from build123d import *

# Parameters (mm, degrees)
CYLINDER015_R     = 4.5
CYLINDER015_DEPTH = 4.6
CYLINDER014_R     = 6
CYLINDER014_DEPTH = 4.6
CYLINDER013_W     = 6
CYLINDER013_H     = 5
CYLINDER013_ANGLE = 39
CYLINDER012_W     = 7
CYLINDER012_H     = 5
CYLINDER012_ANGLE = 39
CHAMFER007_SIZE   = 0.2
ARRAY001_COUNT    = 9


with BuildPart() as cilindro011:
    # Cylinder015 → Cylinder015 (new body)
    with BuildSketch(Plane.XY.offset(0.2)):
        Circle(CYLINDER015_R)
    extrude(amount=CYLINDER015_DEPTH)


with BuildPart() as cut007:
    # Cylinder014 → Cylinder014 (new body)
    with BuildSketch(Plane.XY.offset(0.2)):
        Circle(CYLINDER014_R)
    extrude(amount=CYLINDER014_DEPTH)

    # Cut007: cut Cilindro011
    add(cilindro011.part, mode=Mode.SUBTRACT)


with BuildPart() as cilindro009:
    # Cylinder013 → Cylinder013 (revolve)
    with BuildSketch(Plane.XZ):
        with Locations((3, 2.5)):
            Rectangle(CYLINDER013_W, CYLINDER013_H)
    revolve(axis=Axis((0, 0, 0), (0, 0, 1)), revolution_arc=CYLINDER013_ANGLE)


with BuildPart() as obj1:
    # Cylinder012 → Cylinder012 (revolve)
    with BuildSketch(Plane.XZ):
        with Locations((3.5, 2.5)):
            Rectangle(CYLINDER012_W, CYLINDER012_H)
    revolve(axis=Axis((0, 0, 0), (0, 0, 1)), revolution_arc=CYLINDER012_ANGLE)

    # Cut006: cut Cilindro009
    add(cilindro009.part, mode=Mode.SUBTRACT)

    # Chamfer007
    chamfer007_edges = [obj1.edges().sort_by_distance(p)[0] for p in [
        (5.655849, 2.002841, 5),
        (5.655849, 2.002841, 0),
    ]]
    chamfer(chamfer007_edges, length=CHAMFER007_SIZE)

    # Array001: obj1 ×9 about axis
    array001_axis = Axis((0, 0, 0), (0, 0, 1))


with BuildPart() as obj1_1:
    add(obj1.part)
    for i in range(1, ARRAY001_COUNT):
        add(obj1.part.rotate(array001_axis, i * 360 / ARRAY001_COUNT))

    # Fusion001: union Cut007
    add(cut007.part)


solid = obj1_1.part
Could you check a few things on this model? Use its own coordinates, in mm. Round coordinates to 2 decimals unless told otherwise and drop trailing zeros. Write each loop counter-clockwise with the first axis right and the second up, starting at its lowest first coordinate (ties: lowest second). Pieces come first, ordered by that corner, then holes. Notation, with made-up numbers: (49.5, -7) - (59.5, -7) arc R25 cw to (59.5, 25) - close; hole circle Ø5 at (25, 36). An arc over 180 degrees is marked (long way). Use a Markdown table: item, result.
Q1. I want a section at A-A (x = 0). List the corners of the cut face in (y, z) for me, plus the area to 3 significant figures.
Output values:
| item | result |
|---|---|
| outline | (-7, 0) - (-6.2, 0) - (-6, 0.2) - (-4.5, 0.2) - (-4.5, 4.8) - (-6, 4.8) - (-6.2, 5) - (-7, 5) - close; (4.5, 0.2) - (6, 0.2) - (6.2, 0) - (7, 0) - (7, 5) - (6.2, 5) - (6, 4.8) - (4.5, 4.8) - close |
| area | 23.7 mm2 |
Q2. Please list where these lines run through material, in increasing order: L1, parallel to Y at x = 0, z = 1.65; L2, parallel to Z at x = 0.75, y = 4.75; L3, parallel to Y at x = -3.75, z = 2.7.
Output values:
| item | result |
|---|---|
| L1 | -7 to -4.5, 4.5 to 7 |
| L2 | 0.2 to 4.8 |
| L3 | -5.91 to -2.49, 2.49 to 5.91 |
Q3. For pin 1 (0.5 mm diameter, centred on x = 6.5, z = 2, fed in from -Y); pin 2 (2 mm diameter, centred on x = -3.5, z = 3, fed in from +Y); pin 3 (4 mm diameter, centred on x = -3.5, y = -0.5, fed in from +Z), each with a flat end and sliding along its axis, tell me the tip position at first contact or that it passes through.
Output values:
| item | result |
|---|---|
| pin 1 | y = -3.15 |
| pin 2 | y = 6.54 |
| pin 3 | z = 4.8 |
